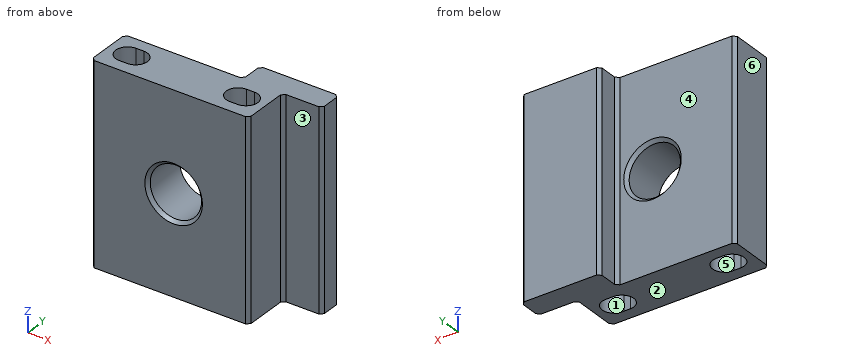
from build123d import *

# Parameters (mm, degrees)
F1_DEPTH = 50
F3_DEPTH = 55
F4_R     = 6.5
F5_DEPTH = 13
F6_SIZE  = 0.8


with BuildPart() as f1:
    # F0 (on Top) → F1 (new body)
    with BuildSketch(Plane.XY):
        Polygon((-32.258, 12), (-32.258, 0), (7.742, 0), (7.742, 12), (17.742, 12), (17.742, 18), (-2.258, 18), (-2.258, 12), align=None)
    extrude(amount=F1_DEPTH)

    # F2 (on face) → F3 (cut)
    with BuildSketch(Plane.XY.offset(50)):
        with BuildLine():
            Line((-25.258, 9), (-27.258, 9))
            ThreePointArc((-27.258, 9), (-30.258, 6), (-27.258, 3))
            Line((-27.258, 3), (-25.596914, 3.019205))
            ThreePointArc((-25.596914, 3.019205), (-22.262805, 5.830271), (-25.258, 9))
        make_face()
        with BuildLine():
            Line((0.742, 3), (2.403086, 3.019205))
            ThreePointArc((2.403086, 3.019205), (5.737195, 5.830271), (2.742, 9))
            Line((2.742, 9), (0.742, 9))
            ThreePointArc((0.742, 9), (-2.258, 6), (0.742, 3))
        make_face()
    extrude(amount=-F3_DEPTH, mode=Mode.SUBTRACT)

    # F4 (on face) → F5 (cut)
    with BuildSketch(Plane.XZ):
        with Locations((-11.308, 25)):
            Circle(F4_R)
    extrude(amount=-F5_DEPTH, mode=Mode.SUBTRACT)

    # F6
    f6_edges = [f1.edges().sort_by_distance(p)[0] for p in [
        (7.742, 0, 25),
        (7.742, 12, 25),
        (17.742, 12, 25),
        (17.742, 18, 25),
        (-32.258, 12, 25),
        (-32.258, 0, 25),
        (-2.258, 12, 25),
        (-2.258, 18, 25),
        (-17.808, 12, 25),
        (-17.808, 0, 25),
    ]]
    chamfer(f6_edges, length=F6_SIZE)


solid = f1.part
The model under review builds one solid part; all positions refer to its coordinate system, in mm. Face numbers are marked on the shaded views. A direction names the side the tool comes from. Round coordinates to 2 decimals unless told otherwise and drop trailing zeros. Write each loop counter-clockwise with the first axis right and the second up, starting at its lowest first coordinate (ties: lowest second). Pieces come first, ordered by that corner, then holes. Notation, with made-up numbers: M 40.25,32.5 L 86.25,32.5 A26 cw 86.25,61.5 Z; hole C 59,-37.75 d7. An arc over 180 degrees is marked long. Use a Markdown table: item, result. Add a question column.
Q1. Machinability: for the marked faces 1, 2 and 3, which of the approach directions +Z, -Z, +X, -X, +Y, -Y give a long, thin tool a straight path to every point of the face, cutting with its end or side? Answer none if there is none.
Q2. The part is to be moulded in two halves that separate along Y. For the marked faces 4, 5 and 6, say which applies: pulls with the +Y half, pulls with the -Y half, needs draft (parallel to the pull), parting line crosses it, or undercut.
Q3. To check wall thickness, follow line 1 (Y direction, x = 2, z = 8); line 2 (X direction, y = 4.25, z = 29); line 3 (X direction, y = 8.5, z = 23). State the ranges of each line that lie inside material, in increasing order.
Q4. We need section C-C, the plane z = 10. State the section outline as (x, y) points.
Q5. Insertion check: pin 1 (6 mm diameter, centred on x = -14, y = 15.5, fed in from -Z); pin 2 (8.5 mm diameter, centred on x = -19.5, z = 16, fed in from +Y); pin 3 (3.5 mm diameter, centred on y = 14.5, z = 17.5, fed in from -X); pin 4 (2.5 mm diameter, centred on x = 11.5, z = 18, fed in from -Y). Each pin has a flat end and moves straight along its axis. Give the tip position at first contact, or say it passes through.
Q6. We need section D-D, the plane x = -24. State the section outline as (y, z) points.
Q7. We need section B-B, the plane y = 6. State the section outline as (x, z) points, plus the area to 3 significant figures.
Q8. We need section A-A, the plane z = 25. Count the separate pieces of the cut face and the enclosed holes in it, plus the area to 3 significant figures.
Findings below:
| question | item | result |
|---|---|---|
| 1 | face 1 | +Z, -Z |
| 1 | face 2 | -Z, +X, -X, +Y, -Y |
| 1 | face 3 | +Z, -Z, +X, -Y |
| 2 | face 4 | pulls with the +Y half |
| 2 | face 5 | undercut |
| 2 | face 6 | needs draft |
| 3 | line 1 | y = 0 to 3.01, 9 to 18 |
| 3 | line 2 | x = -32.26 to -29.69, -22.82 to -16.43, -6.18 to -1.69, 5.18 to 7.74 |
| 3 | line 3 | x = -32.26 to -28.92, -23.6 to -17.49, -5.12 to -0.92, 4.4 to 7.74 |
| 4 | outline | M -32.26,0.8 L -31.46,0 L 6.94,0 L 7.74,0.8 L 7.74,11.2 L 8.54,12 L 16.94,12 L 17.74,12.8 L 17.74,17.2 L 16.94,18 L -1.46,18 L -2.26,17.2 L -2.26,12.8 L -3.06,12 L -31.46,12 L -32.26,11.2 Z; hole M -27.26,3 L -25.6,3.02 A3 ccw long -25.26,9 L -27.26,9 A3 ccw Z; hole M 0.74,3 L 2.4,3.02 A3 ccw long 2.74,9 L 0.74,9 A3 ccw Z |
| 5 | pin 1 | passes through |
| 5 | pin 2 | stops at y = 12 |
| 5 | pin 3 | stops at x = -2.31 |
| 5 | pin 4 | stops at y = 12 |
| 6 | outline | M 0,0 L 3.28,0 L 3.28,50 L 0,50 Z; M 8.72,0 L 12,0 L 12,50 L 8.72,50 Z |
| 7 | outline | M -32.26,0 L -30.26,0 L -30.26,50 L -32.26,50 Z; M -22.26,0 L -2.26,0 L -2.26,50 L -22.26,50 Z; M 5.74,0 L 7.74,0 L 7.74,50 L 5.74,50 Z; hole C -11.31,25 d13 |
| 7 | area | 1,070 mm² |
| 8 | separate pieces | 2 |
| 8 | enclosed holes | 2 |
| 8 | area | 361 mm² |
